from build123d import *

# Parameters (mm, degrees)
ESTRUSIONE_ESTRUSIONE1_DEPTH = 28
ESTRUSIONE_ESTRUSIONE2_DEPTH = 16
SCHIZZO4_W                   = 16
SCHIZZO4_H                   = 50
ESTRUSIONE_ESTRUSIONE3_DEPTH = 6
ESTRUSIONE_ESTRUSIONE4_DEPTH = 22
FORO_PER_VITE_M4_1_D         = 4.5
FORO_PER_VITE_M4_1_DEPTH     = 30
FORO_PER_VITE_M4_1_TIP       = 1.351936393
FORO_PER_VITE_M4_2_D         = 4.5
FORO_PER_VITE_M4_2_DEPTH     = 30
FORO_PER_VITE_M4_2_TIP       = 1.351936393


with BuildPart() as part:
    # Schizzo2 → Estrusione-Estrusione1 (new body)
    with BuildSketch(Plane.XY):
        Polygon((0, 0), (-10, 0), (-10, -25), (-16, -25), (-16, 25), (-10, 25), (-10, 5), (0, 5), (0, 25), (6, 25), (6, -25), (0, -25), align=None)
    extrude(amount=ESTRUSIONE_ESTRUSIONE1_DEPTH)

    # Schizzo3 → Estrusione-Estrusione2 (add)
    with BuildSketch(Plane(origin=(6, 0, 0), x_dir=(0, 0, -1), z_dir=(1, 0, 0))):
        Polygon((-28, 0), (-38, 0), (-38, -25), (-44, -25), (-44, 25), (-38, 25), (-38, 5), (-28, 5), align=None)
    extrude(amount=-ESTRUSIONE_ESTRUSIONE2_DEPTH)

    # Schizzo4 → Estrusione-Estrusione3 (add)
    with BuildSketch(Plane.ZY.offset(10)):
        with Locations((36, 0)):
            Rectangle(SCHIZZO4_W, SCHIZZO4_H)
    extrude(amount=ESTRUSIONE_ESTRUSIONE3_DEPTH)

    # Schizzo5 → Estrusione-Estrusione4 (add)
    with BuildSketch(Plane(origin=(6, 0, 0), x_dir=(0, 0, -1), z_dir=(1, 0, 0))):
        Polygon((-38, -25), (-44, -25), (-44, 25), (-38, 25), (-38, 5), (-28, 5), (-28, 25), (-22, 25), (-22, -25), (-28, -25), (-28, 0), (-38, 0), align=None)
    extrude(amount=ESTRUSIONE_ESTRUSIONE4_DEPTH)

    # Foro per Vite M4-1
    with Locations(Plane.XY.offset(44)):
        with Locations((18, -20)):
            Hole(FORO_PER_VITE_M4_1_D / 2, depth=FORO_PER_VITE_M4_1_DEPTH)
            with Locations((0, 0, -(FORO_PER_VITE_M4_1_DEPTH + FORO_PER_VITE_M4_1_TIP / 2))):  # 118° drill point
                Cone(0, FORO_PER_VITE_M4_1_D / 2, FORO_PER_VITE_M4_1_TIP, mode=Mode.SUBTRACT)

    # Foro per Vite M4-2
    with Locations(Plane.ZY.offset(16)):
        with Locations((10, -20)):
            Hole(FORO_PER_VITE_M4_2_D / 2, depth=FORO_PER_VITE_M4_2_DEPTH)
            with Locations((0, 0, -(FORO_PER_VITE_M4_2_DEPTH + FORO_PER_VITE_M4_2_TIP / 2))):  # 118° drill point
                Cone(0, FORO_PER_VITE_M4_2_D / 2, FORO_PER_VITE_M4_2_TIP, mode=Mode.SUBTRACT)


solid = part.part
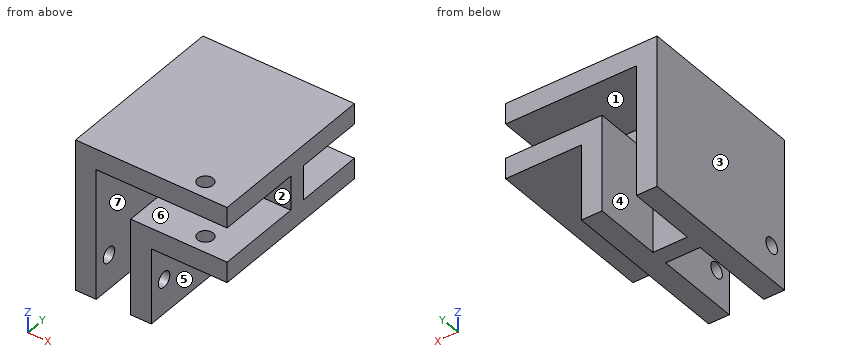
Verification items for the finished model (mm, model axes). Face numbers are marked on the shaded views. A direction names the side the tool comes from. Give positions to 0.01 mm unless a question says otherwise; leave off trailing zeros. Write each loop counter-clockwise with the first axis right and the second up, starting at its lowest first coordinate (ties: lowest second). Pieces come first, ordered by that corner, then holes. Notation, with made-up numbers: (55, 45) - (80, 45) arc R17 ccw to (80, 66) - close; hole circle Ø7 at (60, 33). An arc over 180 degrees is marked (long way). Answer as CSV lines item,"result". Start each with the question number.
1. Sectioned sample at B-B (y = -20). Record the boundary of the cut face in (x, z).
2. Sectioned sample at D-D (z = 29.5). Record the boundary of the cut face in (x, y), then the cut area to 3 significant figures.
3. Draft check along X on the marked faces 1, 2 and 3. Enter one of: pulls with the +X half, pulls with the -X half, needs draft (parallel to the pull), parting line crosses it, or undercut.
4. Depth check by flat-ended pin: pin 1 (2 mm diameter, centred on x = 20.5, y = -14, fed in from -Z); pin 2 (6.5 mm diameter, centred on y = -4, z = 8, fed in from +X). Enter the tip coordinate at first touch or a pass-through.
5. Sectioned sample at A-A (x = 18). Record the boundary of the cut face in (y, z).
6. Thickness scan on line 1 (Y direction, x = 2.95, z = 10); line 2 (X direction, y = -21, z = 14.5); line 3 (Z direction, x = 9, y = -20.5). Record the ranges inside material, lowest first.
7. Sectioned sample at C-C (z = 10). Record the boundary of the cut face in (x, y).
8. Set-up check for the marked faces 4, 5, 6 and 7: record each of +Z, -Z, +X, -X, +Y, -Y from which the full face is reachable in a straight line by a thin tool's end or side.
Derived:
1,outline,"(-16, 0) - (-10, 0) - (-10, 7.75) - (-16, 7.75) - close; (-16, 12.25) - (-10, 12.25) - (-10, 38) - (15.75, 38) - (15.75, 44) - (-16, 44) - close; (0, 0) - (6, 0) - (6, 7.75) - (0, 7.75) - close; (0, 12.25) - (6, 12.25) - (6, 22) - (15.75, 22) - (15.75, 28) - (0, 28) - close; (20.25, 22) - (28, 22) - (28, 28) - (20.25, 28) - close; (20.25, 38) - (28, 38) - (28, 44) - (20.25, 44) - close"
2,outline,"(-16, -25) - (-10, -25) - (-10, 0) - (28, 0) - (28, 5) - (-10, 5) - (-10, 25) - (-16, 25) - close"
2,area,"490 mm²"
3,face 1,"needs draft"
3,face 2,"undercut"
3,face 3,"pulls with the -X half"
4,pin 1,"z = 22"
4,pin 2,"x = 6"
5,outline,"(-25, 22) - (-22.25, 22) - (-22.25, 28) - (-25, 28) - close; (-25, 38) - (-22.25, 38) - (-22.25, 44) - (-25, 44) - close; (-17.75, 22) - (25, 22) - (25, 28) - (5, 28) - (5, 38) - (25, 38) - (25, 44) - (-17.75, 44) - (-17.75, 38) - (0, 38) - (0, 28) - (-17.75, 28) - close"
6,line 1,"-25 to -22.25, -17.75 to 25"
6,line 2,"-16 to -10, 0 to 6"
6,line 3,"22 to 28, 38 to 44"
7,outline,"(-16, -25) - (-10, -25) - (-10, -22.25) - (-16, -22.25) - close; (-16, -17.75) - (-10, -17.75) - (-10, 0) - (0, 0) - (0, -17.75) - (6, -17.75) - (6, 25) - (0, 25) - (0, 5) - (-10, 5) - (-10, 25) - (-16, 25) - close; (0, -25) - (6, -25) - (6, -22.25) - (0, -22.25) - close"
8,face 4,"-Z, +Y"
8,face 5,"-Z, +X, +Y, -Y"
8,face 6,"+X, -Y"
8,face 7,"-Z, -Y"
